Input: part model. Units: mm. Frame: model coordinates. A direction names the side the tool comes from. Coordinates: 2 decimals unless noted, no trailing zeros. Order: outer loops, then holes, each group sorted by start corner. A loop starts at its lowest first (then second) coordinate and runs counter-clockwise, first axis right, second up. Notation, with made-up numbers: (20, 2.25) -> (49, 2.25) arc R27 ccw to (49, 36.25) -> close; hole circle Ø3 at (53.5, 61). An arc over 180 degrees is marked (long way). Answer as CSV lines item,"result".
from build123d import *

# Parameters (mm, degrees)
BEARING_MOUNT_BLOCK_DEPTH                      = 31.0134
BEARING_MOUNT_BLOCK_DEPTH_BACK                 = 5.08
SKETCH1_W                                      = 36.576
SKETCH1_H                                      = 33.274
CBORE_FOR_4_SOCKET_HEAD_CAP_SCREW1_D           = 3.2639
CBORE_FOR_4_SOCKET_HEAD_CAP_SCREW1_DEPTH       = 15.875
CBORE_FOR_4_SOCKET_HEAD_CAP_SCREW1_CBORE_D     = 4.09575
CBORE_FOR_4_SOCKET_HEAD_CAP_SCREW1_CBORE_DEPTH = 4.7625
CBORE_FOR_4_SOCKET_HEAD_CAP_SCREW1_TIP         = 0.980574487
CBORE_FOR_4_SOCKET_HEAD_CAP_SCREW2_D           = 3.2639
CBORE_FOR_4_SOCKET_HEAD_CAP_SCREW2_DEPTH       = 15.875
CBORE_FOR_4_SOCKET_HEAD_CAP_SCREW2_CBORE_D     = 4.09575
CBORE_FOR_4_SOCKET_HEAD_CAP_SCREW2_CBORE_DEPTH = 4.7625
CBORE_FOR_4_SOCKET_HEAD_CAP_SCREW2_TIP         = 0.980574487
SKETCH14_R                                     = 4.0005
ENCODER_MOUNTING_FLANGE_DEPTH                  = 4.7625
ENCODER_MOUNTING_HOLES_3_48_D                  = 1.9939
ENCODER_MOUNTING_HOLES_3_48_DEPTH              = 7.62
ENCODER_MOUNTING_HOLES_3_48_TIP                = 0.599027994
MATERIAL_REDUCTION_CHAMFER_SIZE                = 6.35
MATERIAL_REDUCTION_CHAMFER_2_SIZE              = 6.35
ENCODER_CLEARANCE_CUT_DEPTH                    = 47.706097118
TAPPING_CHAMFER_SIZE                           = 0.762


with BuildPart() as part:
    # Sketch1 → Bearing Mount Block (new, two sides: drawn at the far end of the back side and taken through both)
    with BuildSketch(Plane.XY.offset(-BEARING_MOUNT_BLOCK_DEPTH_BACK)):
        Rectangle(SKETCH1_W, SKETCH1_H)
    extrude(amount=BEARING_MOUNT_BLOCK_DEPTH + BEARING_MOUNT_BLOCK_DEPTH_BACK)

    # CBORE for #4 Socket Head Cap Screw1
    with Locations(Plane(origin=(-14.2875, -16.637, 18.3134), x_dir=(0, 0, -1), z_dir=(0, -1, 0))):
        with Locations((0, 0), (0, 28.575)):
            CounterBoreHole(CBORE_FOR_4_SOCKET_HEAD_CAP_SCREW1_D / 2, CBORE_FOR_4_SOCKET_HEAD_CAP_SCREW1_CBORE_D / 2, CBORE_FOR_4_SOCKET_HEAD_CAP_SCREW1_CBORE_DEPTH, depth=CBORE_FOR_4_SOCKET_HEAD_CAP_SCREW1_DEPTH)
            with Locations((0, 0, -(CBORE_FOR_4_SOCKET_HEAD_CAP_SCREW1_DEPTH + CBORE_FOR_4_SOCKET_HEAD_CAP_SCREW1_TIP / 2))):  # 118° drill point
                Cone(0, CBORE_FOR_4_SOCKET_HEAD_CAP_SCREW1_D / 2, CBORE_FOR_4_SOCKET_HEAD_CAP_SCREW1_TIP, mode=Mode.SUBTRACT)

    # CBORE for #4 Socket Head Cap Screw2
    with Locations(Plane(origin=(0, 16.637, 0), x_dir=(1, 0, 0), z_dir=(0, 1, 0))):
        with Locations((13.5255, 0.3175), (13.5255, -26.2509), (-13.5255, -26.2509), (-13.5255, 0.3175)):
            CounterBoreHole(CBORE_FOR_4_SOCKET_HEAD_CAP_SCREW2_D / 2, CBORE_FOR_4_SOCKET_HEAD_CAP_SCREW2_CBORE_D / 2, CBORE_FOR_4_SOCKET_HEAD_CAP_SCREW2_CBORE_DEPTH, depth=CBORE_FOR_4_SOCKET_HEAD_CAP_SCREW2_DEPTH)
            with Locations((0, 0, -(CBORE_FOR_4_SOCKET_HEAD_CAP_SCREW2_DEPTH + CBORE_FOR_4_SOCKET_HEAD_CAP_SCREW2_TIP / 2))):  # 118° drill point
                Cone(0, CBORE_FOR_4_SOCKET_HEAD_CAP_SCREW2_D / 2, CBORE_FOR_4_SOCKET_HEAD_CAP_SCREW2_TIP, mode=Mode.SUBTRACT)

    # Sketch14 → Encoder Mounting Flange (add)
    with BuildSketch(Plane.XY.offset(14.1859)):
        with BuildLine():
            Line((18.288, -16.637), (9.500261866, -31.703247849))
            ThreePointArc((9.500261866, -31.703247849), (0, -37.1602), (-9.500261866, -31.703247849))
            Line((-9.500261866, -31.703247849), (-18.288, -16.637))
            Line((-18.288, -16.637), (18.288, -16.637))
        make_face()
        with Locations((0, -26.162)):
            Circle(SKETCH14_R, mode=Mode.SUBTRACT)
    extrude(amount=-ENCODER_MOUNTING_FLANGE_DEPTH)

    # Encoder Mounting Holes (#3-48)
    with Locations(Plane(origin=(0, 0, 9.4234), x_dir=(-1, 0, 0), z_dir=(0, 0, -1))):
        with Locations((-3.7211, -32.60713426), (3.7211, -19.71686574), (3.7211, -32.60713426), (-3.7211, -19.71686574)):
            Hole(ENCODER_MOUNTING_HOLES_3_48_D / 2, depth=ENCODER_MOUNTING_HOLES_3_48_DEPTH)
            with Locations((0, 0, -(ENCODER_MOUNTING_HOLES_3_48_DEPTH + ENCODER_MOUNTING_HOLES_3_48_TIP / 2))):  # 118° drill point
                Cone(0, ENCODER_MOUNTING_HOLES_3_48_D / 2, ENCODER_MOUNTING_HOLES_3_48_TIP, mode=Mode.SUBTRACT)

    # Material Reduction Chamfer
    material_reduction_chamfer_edges = [part.edges().sort_by_distance(p)[0] for p in [
        (0, -16.637, 31.0134),
    ]]
    chamfer(material_reduction_chamfer_edges, length=MATERIAL_REDUCTION_CHAMFER_SIZE)

    # Material Reduction Chamfer 2
    material_reduction_chamfer_2_edges = [part.edges().sort_by_distance(p)[0] for p in [
        (0, -16.637, -5.08),
    ]]
    chamfer(material_reduction_chamfer_2_edges, length=MATERIAL_REDUCTION_CHAMFER_2_SIZE)

    # Sketch18 → Encoder Clearance Cut (cut, through all)
    with BuildSketch(Plane(origin=(0, 0, 9.4234), x_dir=(-1, 0, 0), z_dir=(0, 0, -1))):
        with BuildLine():
            Line((12.625716354, -24.7904), (-12.625716354, -24.7904))
            ThreePointArc((-12.625716354, -24.7904), (0, -13.462), (12.625716354, -24.7904))
        make_face()
    extrude(amount=ENCODER_CLEARANCE_CUT_DEPTH, mode=Mode.SUBTRACT)

    # Tapping Chamfer
    tapping_chamfer_edges = [part.edges().sort_by_distance(p)[0] for p in [
        (2.72415, -19.71686574, 9.4234),
        (-4.71805, -32.60713426, 9.4234),
        (-4.71805, -19.71686574, 9.4234),
        (2.72415, -32.60713426, 9.4234),
    ]]
    chamfer(tapping_chamfer_edges, length=TAPPING_CHAMFER_SIZE)


solid = part.part
1. Reachability of faces 4 (the face through (18.288, 0, 13)), 5 (the face through (-13, -16.637, 5)), 6 (the face through (-11.57, 14.29, 25.64)) from +Z, -Z, +X, -X, +Y, -Y: full face, straight path, thin tool, end or side. Return the list, or none.
Findings:
face 4,"+Z, -Z, +X, +Y, -Y"
face 5,"-Z, +X, -X, -Y"
face 6,"+Y"
2. Contact query for flat-ended pins moving along their axis: pin 1 (3.5 mm diameter, centred on x = -13.53, z = 26.25, fed in from -Y); pin 2 (6 mm diameter, centred on y = -23, z = 3.5, fed in from +X); pin 3 (2 mm diameter, centred on x = -13.53, z = -0.32, fed in from +Y); pin 4 (5.5 mm diameter, centred on x = -13.53, z = -0.32, fed in from +Y). Output: stop coordinate, or through.
Findings:
pin 1,"stops at y = -16.64"
pin 2,"passes through"
pin 3,"stops at y = 0.39"
pin 4,"stops at y = 16.64"
3. Cut plane D-D (y = -16). Return the cut outline in (x, z).
Findings:
outline,"(-18.29, 0.63) -> (-7.62, 0.63) -> (-7.62, 9.42) -> (7.62, 9.42) -> (7.62, 0.63) -> (18.29, 0.63) -> (18.29, 25.3) -> (-18.29, 25.3) -> close; hole circle Ø4.1 at (-14.29, 18.31); hole circle Ø4.1 at (14.29, 18.31)"
4. Cut plane C-C (z = 6). Return the cut outline in (x, y), plus the area to 3 significant figures.
Findings:
outline,"(-18.29, -16.64) -> (-8.4, -16.64) arc R12.7 cw to (8.4, -16.64) -> (18.29, -16.64) -> (18.29, 16.64) -> (-18.29, 16.64) -> close"
area,"1,180 mm2"
5. Cut plane B-B (y = 7). Return the cut outline in (x, z), plus the area to 3 significant figures.
Findings:
outline,"(-18.29, -5.08) -> (18.29, -5.08) -> (18.29, 31.01) -> (-18.29, 31.01) -> close; hole circle Ø3.26 at (-13.53, -0.32); hole circle Ø3.26 at (-13.53, 26.25); hole circle Ø3.26 at (13.53, -0.32); hole circle Ø3.26 at (13.53, 26.25)"
area,"1,290 mm2"
6. Ray query, line 1 along Y through (x, z) = (13.5, 3); line 2 along Z through (x, y) = (8.5, -25); line 3 along Y through (x, z) = (1, 11.5). Return the intervals inside material, ascending.
Findings:
line 1,"y = -16.64 to 16.64"
line 2,"z = 9.42 to 14.19"
line 3,"y = -37.11 to -30.04, -22.29 to 16.64"
7. Mould query, pull axis Z, two halves, no side actions, for faces 1 (the face through (-0.3, -13.4, 27.9)), 2 (the face through (13.464, -0.048, 26.528)), 3 (the face through (0.16, -37.16, 11.84)). Classes: released by +Z, released by -Z, zero draft, split by the parting line, or undercut.
Findings:
face 1,"released by +Z"
face 2,"undercut"
face 3,"zero draft"
8. Cut plane A-A (x = 0). Return the cut outline in (y, z) (1 decimal).
Findings:
outline,"(-37.2, 9.4) -> (-30.2, 9.4) -> (-30.2, 14.2) -> (-37.2, 14.2) -> close; (-22.2, 9.4) -> (-13.5, 9.4) -> (-13.5, -1.9) -> (-10.3, -5.1) -> (16.6, -5.1) -> (16.6, 31) -> (-10.3, 31) -> (-16.6, 24.7) -> (-16.6, 14.2) -> (-22.2, 14.2) -> close"
